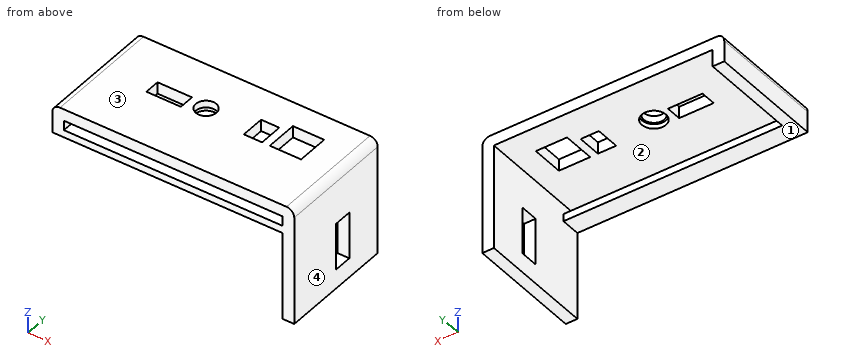
Autodesk Inventor part; units mm, degrees
ref_plane "YZ Plane" through (0, 0, 0) normal (1, 0, 0) x (0, 1, 0)
ref_plane "XZ Plane" through (0, 0, 0) normal (0, 1, 0) x (-1, 0, 0)
ref_plane "XY Plane" through (0, 0, 0) normal (0, 0, 1) x (1, 0, 0)
sketch "Sketch1" plane through (0, 0, 0) normal (0, 1, 0) x (-1, 0, 0)
  line L0 (-31.2, -81) -> (31.2, -81)
  line L1 (31.2, -81) -> (31.2, 81)
  line L2 (31.2, 81) -> (-31.2, 81)
  line L3 (-31.2, 81) -> (-31.2, -81)
  line L4 (-31.2, -81) -> (31.2, 81) construction
  line L5 (31.2, -81) -> (-31.2, 81) construction
  point P0 (0, 0)
  dimension "d0" = 62.4
  dimension "d1" = 162
extrude "Extrusion1" add sketch "Sketch1" along normal blind 3
sketch "Sketch2" plane through (0, 3, 0) normal (0, 1, 0) x (1, 0, 0)
  line L0 (-31.2, 81) -> (-31.2, -81)
  line L1 (-31.2, -81) -> (31.2, -81)
  line L2 (31.2, -81) -> (31.2, 81)
  line L3 (31.2, 81) -> (-31.2, 81)
  line L4 (31.2, 81) -> (-31.2, 81)
  line L5 (-31.2, 81) -> (-31.2, -81)
  line L6 (-31.2, -81) -> (31.2, -81)
  line L7 (31.2, -81) -> (31.2, 81)
  line L8 (31.2, 81) -> (-31.2, -81) construction
  line L9 (-31.2, 81) -> (31.2, -81) construction
  line L10 (28.2, 78) -> (-28.2, 78)
  line L11 (-28.2, 78) -> (-28.2, -78)
  line L12 (-28.2, -78) -> (28.2, -78)
  line L13 (28.2, -78) -> (28.2, 78)
  line L14 (28.2, 78) -> (-28.2, -78) construction
  line L15 (-28.2, 78) -> (28.2, -78) construction
  point P0 (0, 0)
  dimension "d4" = 0
  dimension "d5" = 0
  dimension "d6" = 3
  dimension "d7" = 3
extrude "Extrusion2" add sketch "Sketch2" along normal blind 30
fillet "Fillet1" radius 2 4 edges at (31.2, 16.5, 81) (31.2, 16.5, -81) (-31.2, 16.5, 81) (-31.2, 16.5, -81)
sketch "Sketch9" plane through (0, 3, 0) normal (0, 1, 0) x (1, 0, 0)
  line L0 (28.2, 78) -> (-28.2, 78)
  line L1 (-28.2, 78) -> (-28.2, -78)
  line L2 (-28.2, -78) -> (28.2, -78)
  line L3 (28.2, -78) -> (28.2, 78)
  line L4 (-28.2, -75.5) -> (28.2, -75.5)
  line L5 (28.2, -75.5) -> (28.2, -73.6)
  line L6 (28.2, -73.6) -> (-28.2, -73.6)
  line L7 (-28.2, -73.6) -> (-28.2, -75.5)
  line L8 (-28.2, 78) -> (-28.2, -78)
  line L9 (-28.2, 32.8) -> (28.2, 32.8)
  line L10 (28.2, 32.8) -> (28.2, 34.7)
  line L11 (28.2, 34.7) -> (-28.2, 34.7)
  line L12 (-28.2, 34.7) -> (-28.2, 32.8)
  line L13 (-28.2, 34.7) -> (-11, 34.7)
  line L14 (-11, 34.7) -> (-11, 32.8)
  line L15 (-11, 32.8) -> (-28.2, 32.8)
  line L16 (-28.2, 32.8) -> (-28.2, 34.7)
  line L17 (28.2, 39.1) -> (-11, 39.1)
  line L18 (-11, 39.1) -> (-11, 37.2)
  line L19 (-11, 37.2) -> (28.2, 37.2)
  line L20 (28.2, 37.2) -> (28.2, 39.1)
  line L21 (-11, 37.2) -> (-9, 37.2)
  line L22 (-9, 37.2) -> (-9, 34.7)
  line L23 (-9, 34.7) -> (-11, 34.7)
  line L24 (-11, 34.7) -> (-11, 37.2)
  point P0 (0, 0)
  point P1 (28.2, 14.2)
  point P2 (-28.2, 34.7)
  point P3 (28.2, 32.8)
  point P4 (-28.2, -73.6)
  point P5 (-11, 34.7)
  point P6 (28.2, 37.2)
  dimension "d79" = 1.9
  dimension "d80" = 2.5
  dimension "d81" = 1.9
  dimension "d82" = 106.4
  dimension "d87" = 17.2
  dimension "d163" = 1.9
  dimension "d164" = 2.5
  dimension "d165" = 17.2
  dimension "d166" = 2
extrude "Extrusion9" add sketch "Sketch9" along normal blind 5 contours L3 L19 L18 L17 | L24 L19 L22 L11 | L11 L3 L9 L14 | L6 L3 L4 L1
sketch "Sketch10" plane through (0, 3, 0) normal (0, 1, 0) x (1, 0, 0)
  line L0 (-28.2, -73.6) -> (28.2, -73.6)
  line L1 (28.2, -73.6) -> (28.2, 32.8)
  line L2 (28.2, 32.8) -> (-11, 32.8)
  line L3 (-9, 34.7) -> (28.2, 34.7)
  line L4 (28.2, 34.7) -> (28.2, 37.2)
  line L5 (28.2, 78) -> (-28.2, 78)
  line L6 (-28.2, 78) -> (-28.2, -73.6)
  line L7 (-28.2, 37.1) -> (28.2, 37.1)
  line L8 (-28.2, 70.3) -> (-28.2, 37.1)
  line L9 (-28.2, 37.1) -> (28.2, 37.1)
  line L10 (28.2, 37.1) -> (28.2, 39.1)
  line L11 (28.2, 39.1) -> (-28.2, 39.1)
  line L12 (-28.2, 39.1) -> (-28.2, 37.1)
  line L13 (28.2, 34.7) -> (28.2, 78)
  line L14 (-28.2, 39.1) -> (28.2, 39.1)
  line L15 (28.2, 39.1) -> (28.2, 75.6)
  line L16 (28.2, 75.6) -> (-23, 75.6)
  line L17 (-23, 75.6) -> (28.2, 75.6)
  line L18 (28.2, 75.6) -> (28.2, 68)
  line L19 (-23, 73.5) -> (-23, 75.6)
  line L20 (28.2, 39.1) -> (26.2, 39.1)
  line L21 (26.2, 39.1) -> (26.2, 75.6)
  line L22 (26.2, 75.6) -> (28.2, 75.6)
  line L23 (28.2, 75.6) -> (28.2, 39.1)
  line L24 (26.2, 39.1) -> (9.6, 39.1)
  line L25 (9.6, 39.1) -> (9.6, 75.6)
  line L26 (9.6, 75.6) -> (26.2, 75.6)
  line L27 (26.2, 75.6) -> (26.2, 39.1)
  line L28 (9.6, 39.1) -> (7.6, 39.1)
  line L29 (7.6, 39.1) -> (7.6, 75.6)
  line L30 (7.6, 75.6) -> (9.6, 75.6)
  line L31 (9.6, 75.6) -> (9.6, 39.1)
  line L32 (7.6, 39.1) -> (-9, 39.1)
  line L33 (-9, 39.1) -> (-9, 75.6)
  line L34 (-9, 75.6) -> (7.6, 75.6)
  line L35 (7.6, 75.6) -> (7.6, 39.1)
  line L36 (-9, 39.1) -> (-11, 39.1)
  line L37 (-11, 39.1) -> (-11, 75.6)
  line L38 (-11, 75.6) -> (-9, 75.6)
  line L39 (-9, 75.6) -> (-9, 39.1)
  line L40 (-23, 75.6) -> (-21.5, 75.6)
  line L41 (-21.5, 75.6) -> (-21.5, 39.1)
  line L42 (-21.5, 39.1) -> (-23, 39.1)
  line L43 (-23, 39.1) -> (-23, 75.6)
  line L44 (-11, 39.2) -> (-11, 57)
  line L45 (-11, 57) -> (-21.5, 57)
  line L46 (-21.5, 57) -> (-21.5, 39.1)
  line L47 (-11, 39.1) -> (28.2, 39.1)
  line L48 (28.2, 39.1) -> (28.2, 78)
  line L49 (-11, 32.8) -> (-11, 39.1)
  line L50 (28.2, 37.2) -> (-9, 37.2)
  line L51 (-9, 37.2) -> (-9, 34.7)
  line L52 (28.2, -75.5) -> (-28.2, -75.5)
  line L53 (-28.2, -75.5) -> (-28.2, -78)
  line L54 (-28.2, -78) -> (28.2, -78)
  line L55 (28.2, -78) -> (28.2, -75.5)
  line L56 (-11, 39.2) -> (-11, 37.1)
  line L57 (-11, 55) -> (-23, 55)
  line L58 (-11, 39.2) -> (-11, 32.8)
  line L59 (-11, 32.8) -> (-11, 32.8)
  line L60 (-11, 32.8) -> (-11, 39.2)
  line L61 (-23, 55) -> (-28.2, 55)
  point P0 (0, 0)
  point P1 (28.2, 37.1)
  point P2 (-9, 39.1)
  point P3 (-11, 39.1)
  point P4 (-21.5, 39.1)
  point P5 (-21.5, 57)
  point P6 (28.2, 37.2)
  point P7 (-11, 37.1)
  point P8 (28.2, 39.1)
  point P9 (-25.2, 72.6)
  point P10 (-11, 39.2)
  point P11 (-11, 39.1)
  point P12 (-11, 55)
  point P13 (-21.5, 75.6)
  point P14 (-25.2, 52)
  point P15 (-11, 37.1)
  point P16 (28.2, 39.1)
  point P17 (-11, 37.1)
  point P18 (-21.5, 55)
  point P19 (-11, 39.1)
  point P20 (-10.1, 32.8)
  point P21 (28.2, 39.1)
  point P22 (-11, 39.1)
  point P23 (-9, 39.1)
  point P24 (-11, 32.8)
  dimension "d90" = 2
  dimension "d91" = 36.5
  dimension "d93" = 2
  dimension "d94" = 16.6
  dimension "d95" = 2
  dimension "d96" = 16.6
  dimension "d97" = 2
  dimension "d98" = 1.5
  dimension "d167" = 2.4
  dimension "d172" = 18.6
  dimension "d173" = 2
  dimension "d174" = 10.5
extrude "Extrusion10" add sketch "Sketch10" along normal blind 1 contours L6 L5 L13 L16 L19 L43 L61 | L37 L16 L33 L11 | L43 L19 L16 L41 L57 | L41 L45 L37 L57 | L29 L16 L25 L11 | L11 L21 L16 L13
sketch "Sketch11" plane through (-23.2, 5, 81) normal (0, 0, 1) x (1, 0, 0)
  line L0 (-6, 28) -> (52.4, 28)
  line L1 (5.5, 13) -> (14.4, 13)
  line L2 (14.4, 13) -> (14.4, 17)
  line L3 (14.4, 17) -> (5.5, 17)
  line L4 (5.5, 17) -> (5.5, 13)
  line L5 (45.4, 13) -> (37.34, 13)
  line L6 (37.34, 13) -> (37.34, 21.3)
  line L7 (37.34, 21.3) -> (45.4, 21.3)
  line L8 (45.4, 21.3) -> (45.4, 13)
  circle A0 centre (19, 15.65) radius 2.65
  line L9 (48.4, 0) -> (48.4, 30)
  line L10 (52.4, 28) -> (52.4, -5)
  line L11 (-6, -5) -> (-6, 28)
  line L12 (-6, -5) -> (52.4, -5)
  line L13 (54.4, -5) -> (54.4, 28)
  line L14 (-8, 28) -> (-8, -5)
  line L15 (30.64, 13) -> (35.34, 13)
  line L16 (35.34, 13) -> (35.34, 19.2)
  line L17 (35.34, 19.2) -> (30.64, 19.2)
  line L18 (30.64, 19.2) -> (30.64, 13)
  point P0 (23.2, -5)
  point P1 (46.4, 0)
  point P2 (0, 0)
  dimension "d110" = 8.9
  dimension "d111" = 4
  dimension "d112" = 8.06
  dimension "d113" = 8.3
  dimension "d114" = 5.3
  dimension "d149" = 9
  dimension "d150" = 13.5
  dimension "d151" = 27
  dimension "d152" = 18
  dimension "d153" = 18
  dimension "d154" = 18
  dimension "d168" = 4.7
  dimension "d169" = 6.2
  dimension "d170" = 2
  dimension "d171" = 18
extrude "Extrusion11" cut sketch "Sketch11" against normal blind 3 contours L4 L3 L2 L1 | L5 L6 L7 L8 | A0 | L18 L17 L16 L15
sketch "Sketch12" plane through (28.2, 3, 78) normal (0, 0, -1) x (-1, 0, 0)
  line L0 (14.06, 23.3) -> (14.06, 15)
  line L1 (14.06, 15) -> (6, 15)
  line L2 (6, 15) -> (6, 23.3)
  line L3 (6, 23.3) -> (14.06, 23.3)
  line L4 (37, 19) -> (45.9, 19)
  line L5 (45.9, 19) -> (45.9, 15)
  line L6 (45.9, 15) -> (37, 15)
  line L7 (37, 15) -> (37, 19)
  circle A0 centre (32.4, 17.65) radius 2.65
  line L8 (56.4, 0) -> (0, 0)
  line L9 (56.4, 0) -> (56.4, 30)
  line L10 (0, 30) -> (56.4, 30)
  line L11 (0, 0) -> (0, 30)
  circle A1 centre (32.4, 17.65) radius 3.1
  point P0 (28.2, -3)
  dimension "d128" = 6.2
extrude "Extrusion12" cut sketch "Sketch12" against normal blind 1.2 contours A1
sketch "Sketch13" plane through (23.2, 5, -81) normal (0, 0, -1) x (-1, 0, 0)
  line L0 (-5, 18) -> (51.4, 18)
  line L1 (51.4, 18) -> (51.4, 8.4)
  line L2 (51.4, 8.4) -> (-5, 8.4)
  line L3 (-5, 8.4) -> (-5, 18)
  line L4 (54.4, -5) -> (54.4, 28)
  line L5 (-8, 28) -> (-8, -5)
  line L6 (-6, -5) -> (52.4, -5)
  point P0 (23.2, -5)
  point P1 (51.4, 0)
  point P2 (-5, 0)
  point P3 (-8, -5)
  point P4 (54.4, 11.5)
  point P5 (51.4, 13.2)
  dimension "d131" = 9.6
  dimension "d146" = 3
  dimension "d147" = 3
  dimension "d156" = 23
extrude "Extrusion13" add sketch "Sketch13" along normal blind 6
sketch "Sketch14" plane through (-28.2, 13.4, -81) normal (-1, 0, 0) x (0, 0, 1)
  line L0 (0, 9.6) -> (0, 0)
  line L1 (0, 9.6) -> (-6, 9.6)
  line L2 (-6, 0) -> (-6, 9.6)
  line L3 (0, 0) -> (-6, 0)
  line L4 (0, 9.6) -> (-3.4, 9.6)
  line L5 (-3.4, 9.6) -> (-3.4, 6.6)
  line L6 (-3.4, 6.6) -> (0, 6.6)
  line L7 (0, 6.6) -> (0, 9.6)
  line L8 (0, 0) -> (-3.4, 0)
  line L9 (-3.4, 0) -> (-3.4, 3)
  line L10 (-3.4, 3) -> (0, 3)
  line L11 (0, 3) -> (0, 0)
  point P0 (81, -13.4)
  point P1 (0, 6.6)
  dimension "d137" = 3.4
  dimension "d138" = 3
  dimension "d139" = 3.4
  dimension "d140" = 3
extrude "Extrusion14" cut sketch "Sketch14" against normal up to surface (56.4 mm away) contours L0 L6 L5 L1 | L0 L3 L9 L10
fillet "Fillet5" radius 1 18 edges at (0, 23, -87) (0, 23, -84.4) (0, 13.4, -87) (0, 13.4, -84.4) (-28.2, 16.4, -82.7) (-28.2, 20, -82.7) (28.2, 16.4, -82.7) (28.2, 20, -82.7) (-28.2, 18.2, -87) (-28.2, 21.5, -84.4) (-28.2, 14.9, -84.4) (-28.2, 23, -85.7) (-28.2, 13.4, -85.7) (28.2, 23, -85.7) (28.2, 13.4, -85.7) (28.2, 14.9, -84.4) (28.2, 18.2, -87) (28.2, 21.5, -84.4)
sketch "Sketch15" plane through (31.2, 0, 79) normal (1, 0, 0) x (0, 0, -1)
  line L0 (11, 22.8) -> (23.1, 22.8)
  line L1 (23.1, 22.8) -> (23.1, 18)
  line L2 (23.1, 18) -> (11, 18)
  line L3 (11, 18) -> (11, 22.8)
  line L4 (-2, 33) -> (-2, 0)
  line L5 (0, 0) -> (158, 0)
  point P0 (79, 0)
  dimension "d157" = 12.1
  dimension "d158" = 4.8
  dimension "d159" = 13
  dimension "d160" = 18
extrude "Extrusion15" cut sketch "Sketch15" against normal blind 3
sketch "Sketch16" plane through (0, 33, 0) normal (0, 1, 0) x (1, 0, 0)
  arc A0 (-29.2, 81) -> (-31.2, 79) centre (-29.2, 79) ccw
  line L0 (-31.2, 79) -> (-31.2, -79)
  arc A1 (-31.2, -79) -> (-29.2, -81) centre (-29.2, -79) ccw
  line L1 (-29.2, -81) -> (29.2, -81)
  arc A2 (29.2, -81) -> (31.2, -79) centre (29.2, -79) ccw
  line L2 (31.2, -79) -> (31.2, 79)
  arc A3 (31.2, 79) -> (29.2, 81) centre (29.2, 79) ccw
  line L3 (29.2, 81) -> (-29.2, 81)
  line L4 (28.2, 78) -> (28.2, -78)
  line L5 (28.2, -78) -> (-28.2, -78)
  line L6 (-28.2, -78) -> (-28.2, 78)
  line L7 (-28.2, 78) -> (28.2, 78)
  line L8 (31.2, -79) -> (31.2, 79)
  line L9 (31.2, -50.9) -> (-31.2, -50.9)
  line L10 (-31.2, -50.9) -> (-31.2, 149.1)
  line L11 (-31.2, 149.1) -> (31.2, 149.1)
  line L12 (31.2, 149.1) -> (31.2, -50.9)
  line L13 (31.2, -55.9) -> (28.2, -55.9)
  line L14 (-28.2, -73.6) -> (28.2, -73.6)
  line L15 (-31.2, -50.9) -> (-28.2, -50.9)
  line L16 (-28.2, -50.9) -> (-28.2, -73.6)
  line L17 (-28.2, -73.6) -> (-31.2, -73.6)
  line L18 (-31.2, -73.6) -> (-31.2, -50.9)
  point P0 (0, 0)
  point P1 (-28.2, -50.9)
  point P2 (28.2, -50.9)
  dimension "d175" = 200
  dimension "d176" = 5
extrude "Extrusion16" cut sketch "Sketch16" against normal through all contours L3 A3 L2 L9 L4 L7 L6 L0 A0 | A0 L10 L11 L12 A3 L3 | L9 L6 L17 L0 | L6 L7 L4 L9
sketch "Sketch17" plane through (0, 0, 0) normal (0, -1, 0) x (1, 0, 0)
  line L0 (-28.2, 50.9) -> (31.2, 50.9)
  line L1 (31.2, 79) -> (31.2, 50.9)
  arc A0 (31.2, 79) -> (29.2, 81) centre (29.2, 79) ccw
  line L2 (-29.2, 81) -> (29.2, 81)
  arc A1 (-29.2, 81) -> (-31.2, 79) centre (-29.2, 79) ccw
  line L3 (-31.2, 73.6) -> (-31.2, 79)
  line L4 (-31.2, 73.6) -> (-28.2, 73.6)
  line L5 (-28.2, 73.6) -> (-28.2, 50.9)
  point P0 (0, 0)
extrude "Extrusion17" cut sketch "Sketch17" against normal blind 3
properties part number "module_command" material "PC/ABS Plastic"
Input: part model. Units: mm. Frame: model coordinates. Face numbers are marked on the shaded views. Coordinates: 2 decimals unless noted, no trailing zeros. Loops run counter-clockwise (first coordinate to the right, second up) from the corner with the lowest first, then second, coordinate; pieces in that order, holes last. Notation, with made-up numbers: (-4, 40.5) -> (28, 40.5) arc R18 cw to (28, 45.5) -> close; hole circle Ø3 at (81.25, 48). An arc over 180 degrees is marked (long way). Write each question's results on one line, items separated by ' | '. Start each with the question number.
Q1. Section C-C, the plane y = 6.5. Return the cut outline in (x, z).
Q2. Section D-D, the plane y = 20.65. State how many separate pieces and enclosed holes the cut face has, plus the area to 3 significant figures.
Q3. Pull-direction query (Z, two-part tool) for the marked faces 1, 2, 3 and 4; classes: released by +Z, released by -Z, zero draft, split by the parting line, or undercut.
Q4. Section B-B, the plane z = 61. Return the cut outline in (x, y), plus the area to 3 significant figures.
Q5. Section A-A, the plane x = -23. Return the cut outline in (y, z), plus the area to 3 significant figures.
Q6. Pin query (flat end, axial travel): pin 1 (4 mm diameter, centred on y = 12.5, z = 67.5, fed in from -X); pin 2 (1 mm diameter, centred on x = -15.5, y = 20.5, fed in from -Z); pin 3 (7 mm diameter, centred on x = -4.2, y = 20.65, fed in from -Z). Return the tip coordinate at first contact, or that it passes through.
Q7. Ray query, line 1 (Y direction, x = -4, z = 80); line 2 (Y direction, x = -4.2, z = 78.9); line 3 (Z direction, x = 16, y = 4.5). Return the intervals inside material, ascending. Write a range as from..to.
Found:
1) outline: (-31.2, 73.6) -> (28.2, 73.6) -> (28.2, 50.9) -> (31.2, 50.9) -> (31.2, 79) arc R2 ccw to (29.2, 81) -> (-29.2, 81) arc R2 ccw to (-31.2, 79) -> close; hole (-28.2, 75.5) -> (28.2, 75.5) -> (28.2, 78) -> (-28.2, 78) -> close
2) separate pieces: 6 | enclosed holes: 0 | area: 162 mm2
3) face 1: released by -Z | face 2: undercut | face 3: released by +Z | face 4: zero draft
4) outline: (28.2, 3) -> (31.2, 3) -> (31.2, 18) -> (28.2, 18) -> close; (28.2, 22.8) -> (31.2, 22.8) -> (31.2, 33) -> (28.2, 33) -> close | area: 75.6 mm2
5) outline: (3, 73.6) -> (8, 73.6) -> (8, 75.5) -> (3, 75.5) -> close; (3, 78) -> (33, 78) -> (33, 81) -> (3, 81) -> close | area: 99.5 mm2
6) pin 1: x = 28.2 | pin 2: through | pin 3: z = 78
7) line 1: 3..18.01, 23.29..33 | line 2: 3..17.55, 23.75..33 | line 3: 73.6..75.5, 78..81
